Autodesk Inventor part; units mm, degrees
ref_plane "YZ Plane" through (0, 0, 0) normal (1, 0, 0) x (0, 1, 0)
ref_plane "XZ Plane" through (0, 0, 0) normal (0, 1, 0) x (-1, 0, 0)
ref_plane "XY Plane" through (0, 0, 0) normal (0, 0, 1) x (1, 0, 0)
sketch "Skizze1" plane through (0, 0, 0) normal (0, 1, 0) x (-1, 0, 0)
  line L0 (4.9, 0) -> (-4.9, 0)
  line L1 (-4.9, 0) -> (-7.5, 2.6)
  line L2 (-7.5, 2.6) -> (-7.5, 17)
  line L3 (-7.5, 17) -> (7.5, 17)
  line L4 (7.5, 17) -> (7.5, 2.6)
  line L5 (7.5, 2.6) -> (4.9, 0)
  line L6 (0, -3.4) -> (0, 20.4)
  circle A0 centre (5.5, 3.6) radius 1.05
  circle A1 centre (-5.5, 3.6) radius 1.05
  point P0 (0, 0)
  dimension "d0" = 45
  dimension "d1" = 15
  dimension "d2" = 2.6
  dimension "d3" = 17
  dimension "d4" = 2.1
  dimension "d5" = 2.1
  dimension "d6" = 11
  dimension "d7" = 1
extrude "Extrusion1" add sketch "Skizze1" along normal blind 1
fillet "Rundung1" [suppressed]
sketch "Skizze2" plane through (0, 0, 0) normal (0, 1, 0) x (-1, 0, 0)
  line L0 (5.25, 15) -> (-5.25, 15) construction
  line L1 (0, -3) -> (0, 18)
  line L2 (-7.35, 0) -> (7.35, 0)
  point P0 (0, 0)
  point P1 (1.75, 15)
  point P2 (-1.75, 15)
  dimension "d11" = 3.5
  dimension "d12" = 3.5
  dimension "d13" = 15
hole "Bohrung1" at (1.75, 0, 15) at (-1.75, 0, 15) at (-5.25, 0, 15) at (5.25, 0, 15) direction (0, 1, 0) diameter 1 end through all
properties part number "Encoderplatine" material "Phenolharz"
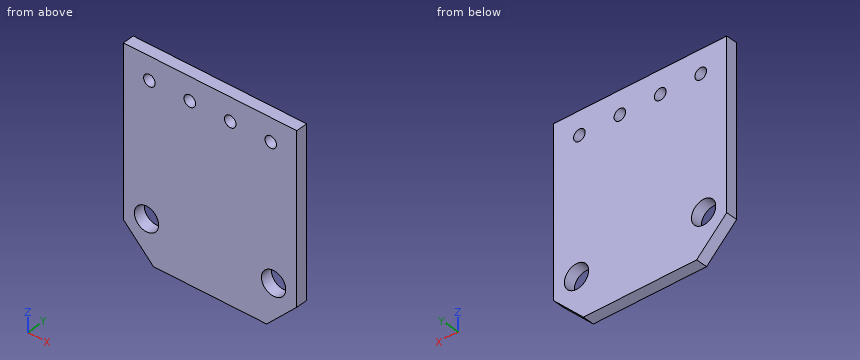
For this review, take the finished solid that the model builds, in its own axes (mm). Round coordinates to 2 decimals unless told otherwise and drop trailing zeros. Write each loop counter-clockwise with the first axis right and the second up, starting at its lowest first coordinate (ties: lowest second). Pieces come first, ordered by that corner, then holes. Notation, with made-up numbers: (-29, -36) - (-14, -36) arc R14 ccw to (-14, -22) - close; hole circle Ø10 at (38.5, -17). An arc over 180 degrees is marked (long way). Put each result on its own line as item: value.
Q1. We need section B-B (y = 0.75). Give the boundary of the cut face in (x, z), and give its area (3 significant figures).
Solved:
outline: (-7.5, 2.6) - (-4.9, 0) - (4.9, 0) - (7.5, 2.6) - (7.5, 17) - (-7.5, 17) - close; hole circle Ø2.1 at (-5.5, 3.6); hole circle Ø1 at (-5.25, 15); hole circle Ø1 at (-1.75, 15); hole circle Ø1 at (1.75, 15); hole circle Ø2.1 at (5.5, 3.6); hole circle Ø1 at (5.25, 15)
area: 238 mm2
Q2. We need section A-A (x = -1.75). Give the boundary of the cut face in (y, z), and give its area (3 significant figures).
Solved:
outline: (0, 0) - (1, 0) - (1, 14.5) - (0, 14.5) - close; (0, 15.5) - (1, 15.5) - (1, 17) - (0, 17) - close
area: 16.0 mm2
Q3. We need section D-D (x = 5.5). Give the boundary of the cut face in (y, z).
Solved:
outline: (0, 0.6) - (1, 0.6) - (1, 2.55) - (0, 2.55) - close; (0, 4.65) - (1, 4.65) - (1, 14.57) - (0, 14.57) - close; (0, 15.43) - (1, 15.43) - (1, 17) - (0, 17) - close
Q4. We need section C-C (z = 3.6). Give the boundary of the cut face in (x, y), and give its area (3 significant figures).
Solved:
outline: (-7.5, 0) - (-6.55, 0) - (-6.55, 1) - (-7.5, 1) - close; (-4.45, 0) - (4.45, 0) - (4.45, 1) - (-4.45, 1) - close; (6.55, 0) - (7.5, 0) - (7.5, 1) - (6.55, 1) - close
area: 10.8 mm2
Q5. Wall thickness on probe 1 along X at (y, z) = (0.3, 15); probe 2 along Z at (x, y) = (1.75, 0.45); probe 3 along Z at (x, y) = (5.25, 0.8): over which ranges is each line inside the solid? List them lowest first.
Solved:
probe 1: x = -7.5 to -5.75, -4.75 to -2.25, -1.25 to 1.25, 2.25 to 4.75, 5.75 to 7.5
probe 2: z = 0 to 14.5, 15.5 to 17
probe 3: z = 0.35 to 2.58, 4.62 to 14.5, 15.5 to 17
Q6. Insertion check: pin 1 Ø1.7 at (x, z) = (-5.5, 3.6) entering from -Y. The pin has a flat end and moves straight along its axis. Give the tip position at first contact, or say it passes through.
Solved:
pin 1: passes through
